```python
from build123d import *

# Parameters (mm, degrees)
SKETCH1_W           = 138
SKETCH1_H           = 95
BOSS_EXTRUDE1_DEPTH = 15
SKETCH2_W           = 128
SKETCH2_H           = 86
CUT_EXTRUDE1_DEPTH  = 7
SNAP_START          = 64.5
SNAP_HOOK2_DEPTH    = 2
SNAP_HOOK2_2_DEPTH  = 2
FILLET1_R           = 1
FILLET2_R           = 0.5
SCALE1_SCALE        = 0.4


with BuildPart() as part:
    # Sketch1 → Boss-Extrude1 (new body)
    with BuildSketch(Plane(origin=(0, 0, 0), x_dir=(1, 0, 0), z_dir=(0, 1, 0))):
        Rectangle(SKETCH1_W, SKETCH1_H)
    extrude(amount=BOSS_EXTRUDE1_DEPTH)

    # Sketch2 → Cut-Extrude1 (cut)
    with BuildSketch(Plane(origin=(0, 15, 0), x_dir=(1, 0, 0), z_dir=(0, 1, 0))):
        Rectangle(SKETCH2_W, SKETCH2_H)
    extrude(amount=-CUT_EXTRUDE1_DEPTH, mode=Mode.SUBTRACT)



with BuildPart() as body_2:
    # Snap Hook2: read off the stored shape, not the designer's step
    # Snap Hook2 outline → Snap Hook2 (new body)
    with BuildSketch(Plane.YZ.offset(SNAP_START)):
        Polygon((21, -2), (21, 2), (18, 2.157223338), (18, -2.157223338), align=None)
    snap_hook2 = extrude(amount=SNAP_HOOK2_DEPTH)


with BuildPart() as part_1:
    add(part.part)

    add(body_2.part)  # Snap Hook2 2 merges body 2
    # Snap Hook2 2 outline → Snap Hook2 2 (add)
    with BuildSketch(Plane.YZ.offset(SNAP_START)):
        Polygon((18, -2.157223338), (18, 2.157223338), (15, 2.314446676), (15, -2.314446676), align=None)
    snap_hook2_2 = extrude(amount=SNAP_HOOK2_2_DEPTH)

    # Snap Hook2 3: loft between two sections, ruled curve by curve
    snap_hook2_3_from = [
        Edge.make_line((66.5, 21, -2), (66.5, 21, 2)),
        Edge.make_line((66.5, 18, 2.157223338), (66.5, 18, -2.157223338)),
        Edge.make_line((66.5, 18, 2.157223338), (66.5, 21, 2)),
        Edge.make_line((66.5, 18, -2.157223338), (66.5, 21, -2)),
    ]
    snap_hook2_3_to = [
        Edge.make_line((68.5, 19, -2.104815559), (68.5, 19, 2.104815559)),
        Edge.make_line((68.5, 18, 2.157223338), (68.5, 18, -2.157223338)),
        Edge.make_line((68.5, 18, 2.157223338), (68.5, 19, 2.104815559)),
        Edge.make_line((68.5, 18, -2.157223338), (68.5, 19, -2.104815559)),
    ]
    snap_hook2_3 = Solid(Shell([*[Face.make_surface_from_curves(snap_hook2_3_from[k], snap_hook2_3_to[k]) for k in range(4)], Face(Wire(snap_hook2_3_from)), Face(Wire(snap_hook2_3_to))]))
    add(snap_hook2_3)

    # Fillet1
    fillet1_edges = [part_1.edges().sort_by_distance(p)[0] for p in [
        (64, 11.5, -43),
        (64, 11.5, 43),
        (-64, 11.5, 43),
        (-64, 11.5, -43),
        (-69, 7.5, -47.5),
        (69, 7.5, -47.5),
        (69, 7.5, 47.5),
        (-69, 7.5, 47.5),
    ]]
    fillet(fillet1_edges, radius=FILLET1_R)

    # Mirror1: Snap Hook2, Snap Hook2 2, Snap Hook2 3 across plane
    add(snap_hook2.mirror(Plane(origin=(0, 0, 0), x_dir=(0, 0, 1), z_dir=(1, 0, 0))))
    add(snap_hook2_2.mirror(Plane(origin=(0, 0, 0), x_dir=(0, 0, 1), z_dir=(1, 0, 0))))
    add(snap_hook2_3.mirror(Plane(origin=(0, 0, 0), x_dir=(0, 0, 1), z_dir=(1, 0, 0))))

    # Fillet2
    fillet2_edges = [part_1.edges().sort_by_distance(p)[0] for p in [
        (66.5, 15, 0),
        (64.5, 15, 0),
        (-66.5, 15, 0),
        (-64.5, 15, 0),
    ]]
    fillet(fillet2_edges, radius=FILLET2_R - 0.0001)  # a hair under: the kernel refuses the full size


with BuildPart() as part_2:
    # Scale1: scaled about (0, 4.938102716, 0)
    add(part_1.part.scale(SCALE1_SCALE).moved(Location((0, 2.96286163, 0))))


solid = part_2.part
```
The listing builds one solid part. Answer for the finished solid, in the listing's coordinates (mm). A direction names the side the tool comes from. Give positions to 0.01 mm unless a question says otherwise; leave off trailing zeros. Write each loop counter-clockwise with the first axis right and the second up, starting at its lowest first coordinate (ties: lowest second). Pieces come first, ordered by that corner, then holes. Notation, with made-up numbers: (86, 35) - (133, 35) arc R9 cw to (133, 42) - close; hole circle Ø3 at (-3, -11.75). An arc over 180 degrees is marked (long way). Use one line per item in the form item = value. Start each with the question number.
1) Consider line 1 along X through (y, z) = (8.75, 5); line 2 along Z through (x, y) = (-12, 8); line 3 along Y through (x, z) = (-4, -12). Determine where each line is inside the solid, lowest interval first. Write a range as from..to.
2) Flat-ended cylindrical pins translate along their axes: pin 1 Ø0.8 at (y, z) = (9.5, -0.5) entering from -X; pin 2 Ø0.5 at (y, z) = (11, -0.5) entering from -X; pin 3 Ø1.5 at (y, z) = (10, 0.5) entering from +X. Find the tip coordinate at first contact, or state that the pin passes through.
3) Find section B-B on z = -5.5. Determine the outline of the cut face in (x, y), plus the area to 3 significant figures.
4) A tool of negligible diameter and unlimited length cuts with its end or side. For faces 4 (the face through (0, 6.163, 0)), 5 (the face through (25.8, 10, 0)), 6 (the face through (-26.192, 10.146, -0.864)), from which of +Z, -Z, +X, -X, +Y, -Y can it reach the whole face along a straight path? Write none if from no direction.
5) Find section A-A on x = -1. Determine the outline of the cut face in (y, z), plus the area to 3 significant figures.
6) The mould has two halves that part along Z. Classify faces 1 (the face through (27.6, 6, 0)), 2 (the face through (0, 6, 19)), 3 (the face through (25.6, 8, 0)): pulls with the +Z half, pulls with the -Z half, needs draft (parallel to the pull), parting line crosses it, or undercut.
Geometry results:
q1.line_1 = -27.6..-25.6, 25.6..27.6
q1.line_2 = -19..-17.2, 17.2..19
q1.line_3 = 2.96..6.16
q2.pin_1 = -26.61
q2.pin_2 = -27.21
q2.pin_3 = 27.4
q3.outline = (-27.6, 2.96) - (27.6, 2.96) - (27.6, 8.96) - (25.6, 8.96) - (25.6, 6.16) - (-25.6, 6.16) - (-25.6, 8.96) - (-27.6, 8.96) - close
q3.area = 188 mm2
q4.face_4 = +Y
q4.face_5 = +Z, -Z, +Y
q4.face_6 = -Z, +X, -X, +Y
q5.outline = (2.96, -19) - (8.96, -19) - (8.96, -17.2) - (6.16, -17.2) - (6.16, 17.2) - (8.96, 17.2) - (8.96, 19) - (2.96, 19) - close
q5.area = 132 mm2
q6.face_1 = needs draft
q6.face_2 = pulls with the +Z half
q6.face_3 = undercut
